```python
from build123d import *

# Parameters (mm, degrees)
BOSS_EXTRUDE1_DEPTH = 10
CHAMFER1_SIZE       = 5
CHAMFER3_SIZE       = 1
CHAMFER4_SIZE       = 0.5
CHAMFER5_SIZE       = 0.5


with BuildPart() as part:
    # Sketch1 → Boss-Extrude1 (new body)
    with BuildSketch(Plane(origin=(0, 0, 0), x_dir=(1, 0, 0), z_dir=(0, 1, 0))):
        Polygon((-0.1, 0), (-0.1, 20.1), (3.9, 20.1), (3.9, 28.1), (16.1, 28.1), (16.1, 20.1), (20.1, 20.1), (20.1, 0), (20.1, -0.1), (18.6, -0.1), (18.6, -1.076654702), (25.1, -1.076654702), (25.1, 10), (25.1, 33.1), (-5.1, 33.1), (-5.1, 10), (-5.1, -1.076654702), (1.4, -1.076654702), (1.4, -0.1), (-0.1, -0.1), align=None)
    extrude(amount=BOSS_EXTRUDE1_DEPTH)

    # Chamfer1
    chamfer1_edges = [part.edges().sort_by_distance(p)[0] for p in [
        (-5.1, 5, -33.1),
        (25.1, 5, -33.1),
    ]]
    chamfer(chamfer1_edges, length=CHAMFER1_SIZE)

    # Chamfer3
    chamfer3_edges = [part.edges().sort_by_distance(p)[0] for p in [
        (16.1, 5, -20.1),
        (3.9, 5, -20.1),
        (-5.1, 5, 1.076654702),
        (25.1, 5, 1.076654702),
    ]]
    chamfer(chamfer3_edges, length=CHAMFER3_SIZE)

    # Chamfer4
    chamfer4_edges = [part.edges().sort_by_distance(p)[0] for p in [
        (0.65, 10, 0.1),
        (-0.1, 10, -10),
        (1.4, 10, -20.1),
        (10, 10, -28.1),
        (3.9, 10, -24.6),
        (16.1, 10, -24.6),
        (18.6, 10, -20.1),
        (3.4, 10, -20.6),
        (16.6, 10, -20.6),
        (20.1, 10, -10.05),
        (19.35, 10, 0.1),
    ]]
    chamfer(chamfer4_edges, length=CHAMFER4_SIZE)

    # Chamfer5
    chamfer5_edges = [part.edges().sort_by_distance(p)[0] for p in [
        (18.6, 5, 1.076654702),
        (1.4, 5, 1.076654702),
    ]]
    chamfer(chamfer5_edges, length=CHAMFER5_SIZE)


solid = part.part
```
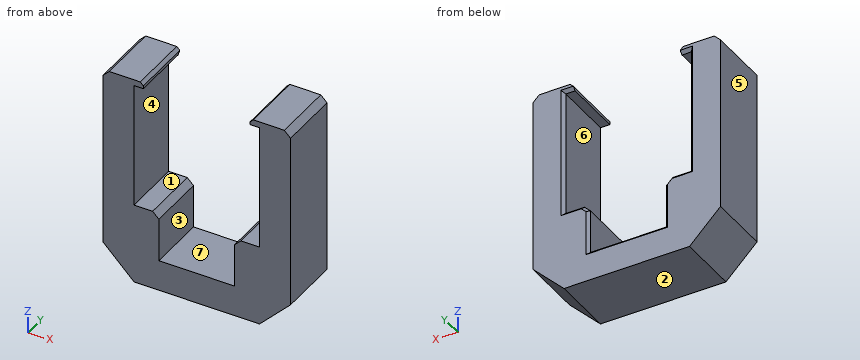
Here's how the part is built. I have some questions about the finished solid (model axes, mm). Face numbers are marked on the shaded views. A direction names the side the tool comes from. Coordinates: 2 decimals unless noted, no trailing zeros. Loops run counter-clockwise (first coordinate to the right, second up) from the corner with the lowest first, then second, coordinate; pieces in that order, holes last. Notation, with made-up numbers: (-5.75, 51) - (49.25, 51) arc R26 cw to (49.25, 87) - close; hole circle Ø9 at (51, 60). An arc over 180 degrees is marked (long way). Return JSON: item names as keys, results as strings. Group by question number.
Item 1: Will these pins go through, and if not, where does the flat tip stop? P1, Ø5, axis at x = 7, y = 3, coming from the +Z side; P2, Ø0.9, axis at x = 2, y = 3, coming from the +Z side.
Item 2: We'd pull the mould along Z, two halves only. Please class the marked faces 1, 2, 3 and 4: +Z half, -Z half, draft (parallel to the pull), parting line (faces both ways), or undercut.
Item 3: If we section it at D-D on z = -30.5: Write out the boundary of the cut face in (x, y), and give its area (3 significant figures).
Item 4: I need wall thicknesses on line 1 (X direction, y = 4.25, z = -2.5); line 2 (Z direction, x = 20, y = 7.25); line 3 (X direction, y = 2.25, z = -27). Which ranges of each line are inside material? Lowest first, please. Write a range as from..to.
Item 5: On a 3-axis mill with a long thin cutter (end or side, diameter ignored), from which of +Z, -Z, +X, -X, +Y, -Y can I reach the whole of each face in a straight line? I mean the marked faces 5, 6 and 7. Say none if no direction works.
Item 6: If we section it at C-C on x = 6: Write out the boundary of the cut face in (y, z), and give its area (3 significant figures).
Item 7: If we section it at B-B on y = 1: Write out the boundary of the cut face in (x, z), and give its area (3 significant figures).
Item 8: If we section it at A-A on z = -10: Write out the boundary of the cut face in (x, y).
Calculated:
{
 "1": {"P1": "stops at z = -28.1", "P2": "stops at z = -20.1"},
 "2": {"face 1": "undercut", "face 2": "-Z half", "face 3": "draft", "face 4": "undercut"},
 "3": {"outline": "(-2.7, 0) - (22.7, 0) - (22.7, 10) - (-2.7, 10) - close", "area": "254 mm^2"},
 "4": {"line 1": "x = -5.1..-0.1, 20.1..25.1", "line 2": "z = -33.1..-20.1, 0.1..1.08", "line 3": "x = -5.1..3.9, 16.1..25.1"},
 "5": {"face 5": "+Z, -Z, -X, +Y, -Y", "face 6": "+Y, -Y", "face 7": "+Z, +Y, -Y"},
 "6": {"outline": "(0, -33.1) - (10, -33.1) - (10, -28.6) - (9.5, -28.1) - (0, -28.1) - close", "area": "49.9 mm^2"},
 "7": {"outline": "(-5.1, -28.1) - (-0.1, -33.1) - (20.1, -33.1) - (25.1, -28.1) - (25.1, 0.08) - (24.1, 1.08) - (19.1, 1.08) - (18.6, 0.58) - (18.6, 0.1) - (20.1, 0.1) - (20.1, -20.1) - (17.1, -20.1) - (16.1, -21.1) - (16.1, -28.1) - (3.9, -28.1) - (3.9, -21.1) - (2.9, -20.1) - (-0.1, -20.1) - (-0.1, 0.1) - (1.4, 0.1) - (1.4, 0.58) - (0.9, 1.08) - (-4.1, 1.08) - (-5.1, 0.08) - close", "area": "482 mm^2"},
 "8": {"outline": "(-5.1, 0) - (-0.1, 0) - (-0.1, 9.5) - (-0.6, 10) - (-5.1, 10) - close; (20.1, 0) - (25.1, 0) - (25.1, 10) - (20.6, 10) - (20.1, 9.5) - close"}
}
